Work out the finished part from the listing and answer in its coordinate system (mm). A direction names the side the tool comes from. Coordinates: 2 decimals unless noted, no trailing zeros. Order: outer loops, then holes, each group sorted by start corner. A loop starts at its lowest first (then second) coordinate and runs counter-clockwise, first axis right, second up.
1. The part is cut by section A-A, the plane y = 2.1. Give the vertices of the cut face in (x, z), then the cut area to 3 significant figures.
2. Flat-ended cylindrical pins translate along their axes: pin 1 Ø1.5 at (x, y) = (-22, 1) entering from -Z; pin 2 Ø1 at (y, z) = (2.5, 5) entering from -X. Find the tip coordinate at first contact, or state that the pin passes through.
3. Determine the mould class of faces 1 (the flat face through (0, 0, 0)), 2 (the cylindrical face through (12.727, 0.616, 13.392)), 3 (the cylindrical face through (23.4, 1.97, 14.92)) for opening direction Z: +Z half, -Z half, draft (parallel to the pull), parting line (faces both ways), or undercut.
4. Find the intervals of material crossed by probe 1 along X at (y, z) = (2.2, -17); probe 2 along X at (y, z) = (3.6, -13.75); probe 3 along Z at (x, y) = (-8.5, 2.85), in increasing order.
5. A tool of negligible diameter and unlimited length cuts with its end or side. For faces 4 (the cylindrical face through (-14.957, 3.754, 13.099)), 5 (the cylindrical face through (-8.141, 0.616, 11.723)), from which of +Z, -Z, +X, -X, +Y, -Y can it reach the whole face along a straight path? Write none if from no direction.
6. The part is cut by section B-B, the plane x = -10. Give the vertices of the cut face in (y, z).
7. The part is cut by section D-D, the plane x = 16. Give the vertices of the cut face in (y, z), then the cut area to 3 significant figures.
8. The part is cut by section C-C, the plane z = 13.75. Give the vertices of the cut face in (x, y).
```python
from build123d import *

# Parameters (mm, degrees)
SKETCH1_R                                      = 27.75
SKETCH1_R_2                                    = 2.75
BOSS_EXTRUDE1_DEPTH                            = 4
CSK_FOR_M5_FLAT_HEAD_MACHINE_SCREW1_AT_2_COUNT = 2
CSK_FOR_M5_FLAT_HEAD_MACHINE_SCREW1_AT_2_PITCH = 27.5
CSK_FOR_M5_FLAT_HEAD_MACHINE_SCREW1_AT_3_COUNT = 2
CSK_FOR_M5_FLAT_HEAD_MACHINE_SCREW1_AT_3_PITCH = 34.003676272
CSK_FOR_M5_FLAT_HEAD_MACHINE_SCREW1_AT_4_COUNT = 2
CSK_FOR_M5_FLAT_HEAD_MACHINE_SCREW1_AT_4_PITCH = 20


with BuildPart() as part:
    # Sketch1 → Boss-Extrude1 (new body)
    with BuildSketch(Plane(origin=(0, 0, 0), x_dir=(1, 0, 0), z_dir=(0, 1, 0))):
        with Locations(Location((0, 0, 0), (0, 0, 270))):
            Circle(SKETCH1_R)
        with Locations(Location((-10, 13.75, 0), (0, 0, 270))):
            Circle(SKETCH1_R_2, mode=Mode.SUBTRACT)
        with Locations(Location((10, 13.75, 0), (0, 0, 270))):
            Circle(SKETCH1_R_2, mode=Mode.SUBTRACT)
        with Locations(Location((10, -13.75, 0), (0, 0, 270))):
            Circle(SKETCH1_R_2, mode=Mode.SUBTRACT)
        with Locations(Location((-10, -13.75, 0), (0, 0, 270))):
            Circle(SKETCH1_R_2, mode=Mode.SUBTRACT)
    extrude(amount=BOSS_EXTRUDE1_DEPTH)

    # Sketch20 → CSK for M5 Flat Head Machine Screw1 (revolve, cut)
    with BuildSketch(Plane(origin=(10, 4, -13.75), x_dir=(0, 0, 1), z_dir=(1, 0, 0))):
        Polygon((0, 0), (0, 4), (2.75, 4), (2.75, 2.75), (5, 0.5), (5, 0), align=None)
    csk_for_m5_flat_head_machine_screw1 = revolve(axis=Axis((10, 10.35, -13.75), (0, -1, 0)), mode=Mode.SUBTRACT)

    # CSK for M5 Flat Head Machine Screw1 at 2: CSK for M5 Flat Head Machine Screw1 ×2
    with Locations(*[(0, 0, i * CSK_FOR_M5_FLAT_HEAD_MACHINE_SCREW1_AT_2_PITCH) for i in range(1, CSK_FOR_M5_FLAT_HEAD_MACHINE_SCREW1_AT_2_COUNT)]):
        add(csk_for_m5_flat_head_machine_screw1, mode=Mode.SUBTRACT)

    # CSK for M5 Flat Head Machine Screw1 at 3: CSK for M5 Flat Head Machine Screw1 ×2
    with Locations(*[Vector(-0.588171697675046, 0, 0.8087360843031888) * (i * CSK_FOR_M5_FLAT_HEAD_MACHINE_SCREW1_AT_3_PITCH) for i in range(1, CSK_FOR_M5_FLAT_HEAD_MACHINE_SCREW1_AT_3_COUNT)]):
        add(csk_for_m5_flat_head_machine_screw1, mode=Mode.SUBTRACT)

    # CSK for M5 Flat Head Machine Screw1 at 4: CSK for M5 Flat Head Machine Screw1 ×2
    with Locations(*[(-i * CSK_FOR_M5_FLAT_HEAD_MACHINE_SCREW1_AT_4_PITCH, 0, 0) for i in range(1, CSK_FOR_M5_FLAT_HEAD_MACHINE_SCREW1_AT_4_COUNT)]):
        add(csk_for_m5_flat_head_machine_screw1, mode=Mode.SUBTRACT)


solid = part.part
```
Geometry says:
1. outline: circle Ø55.5 at (0, 0); hole circle Ø7.2 at (-10, -13.75); hole circle Ø7.2 at (-10, 13.75); hole circle Ø7.2 at (10, -13.75); hole circle Ø7.2 at (10, 13.75)
1. area: 2,260 mm2
2. pin 1: stops at z = -17.85
2. pin 2: stops at x = -27.38
3. face 1: draft
3. face 2: undercut
3. face 3: parting line
4. probe 1: x = -21.93 to -11.77, -8.23 to 8.23, 11.77 to 21.93
4. probe 2: x = -24.1 to -15, -5 to 5, 15 to 24.1
4. probe 3: z = -26.42 to -17.83, -9.67 to 9.67, 17.83 to 26.42
5. face 4: +Y
5. face 5: +Y, -Y
6. outline: (0, -25.89) - (4, -25.89) - (4, -18.75) - (3.5, -18.75) - (1.25, -16.5) - (0, -16.5) - close; (0, -11) - (1.25, -11) - (3.5, -8.75) - (4, -8.75) - (4, 8.75) - (3.5, 8.75) - (1.25, 11) - (0, 11) - close; (0, 16.5) - (1.25, 16.5) - (3.5, 18.75) - (4, 18.75) - (4, 25.89) - (0, 25.89) - close
7. outline: (0, -22.67) - (4, -22.67) - (4, 22.67) - (0, 22.67) - close
7. area: 181 mm2
8. outline: (-24.1, 0) - (-12.75, 0) - (-12.75, 1.25) - (-15, 3.5) - (-15, 4) - (-24.1, 4) - close; (-7.25, 0) - (7.25, 0) - (7.25, 1.25) - (5, 3.5) - (5, 4) - (-5, 4) - (-5, 3.5) - (-7.25, 1.25) - close; (12.75, 0) - (24.1, 0) - (24.1, 4) - (15, 4) - (15, 3.5) - (12.75, 1.25) - close
